Can you work these out from the model? Positions are in its coordinate system, mm. A direction names the side the tool comes from. Give positions to 0.01 mm unless a question says otherwise; leave off trailing zeros. Order: outer loops, then holes, each group sorted by start corner. A loop starts at its lowest first (then second) coordinate and runs counter-clockwise, first axis right, second up. Notation, with made-up numbers: M -21,67 L -7,67 A10 ccw -7,72 Z; hole C 65,34 d11. An arc over 180 degrees is marked long. One line per question, with ' | ' between items. Start each with the question number.
1) If we section it at C-C, the plane z = -25.4: Please give me the cut outline in (x, y) (3 decimals).
2) For faces 1 (the flat face through (84.16, 17.485, -14.31)), 2 (the flat face through (82.55, 12, -38)), which set-ups out of +Z, -Z, +X, -X, +Y, -Y let a thin tool reach every point of the face, with its end or its side?
3) If we section it at A-A, the plane x = 6.35: Please give me the cut outline in (y, z) (3 decimals), plus the area to 3 significant figures.
4) Please list where these lines run through material, in increasing order: line 1 along X through (y, z) = (1.5, -50.8); line 2 along X through (y, z) = (1, -25.4); line 3 along X through (y, z) = (4.5, -28.5) (3 decimals). Write a range as [from, to].
5) I'm going to push flat-ended pins straight in: pin 1 Ø4 at (y, z) = (11.5, -52.5) entering from -X; pin 2 Ø4.5 at (x, z) = (38.1, -25.4) entering from -Y; pin 3 Ø8.5 at (x, z) = (69.85, -50.8) entering from +Y (3 decimals). Where does each tip first touch, or does it pass through?
6) Thinking about a two-plate mould opening in Y: for faces 3 (the cylindrical face through (84.12, 11.27, -23.15)), 4 (the flat face through (84.16, 17.44, -61.935)), 5 (the cylindrical face through (7.151, 1.61, -22.856)), which applies, +Y half, -Y half, draft (parallel to the pull), parting line (faces both ways), or undercut?
7) If we section it at D-D, the plane z = -45: Please give me the cut outline in (x, y) (3 decimals).
8) If we section it at B-B, the plane y = 12.7: Please give me the cut outline in (x, z) (3 decimals).
```python
from build123d import *

# Parameters (mm, degrees)
SKETCH1_W               = 81.788
SKETCH1_H               = 63.5
BOSS_EXTRUDE1_DEPTH     = 3.175
EDGE_FLANGE1_DEPTH      = 63.5
SKETCH6_R               = 2.667
CUT_EXTRUDE1_DEPTH      = 108.856577222
SKETCH7_R               = 2.667
CUT_EXTRUDE2_DEPTH      = 106.875658203
CUT_EXTRUDE3_DEPTH      = 108.856577222
CUT_EXTRUDE3_DEPTH_BACK = 108.856577222
SKETCH8_W               = 104.248957023
SKETCH8_H               = 23.686680931
CHAMFER2_SIZE           = 3.175


# Sheet-metal steps are written as plain solids
with BuildPart() as part:
    # Sketch1 → Boss-Extrude1 (new body)
    with BuildSketch(Plane(origin=(0, 0, 0), x_dir=(1, 0, 0), z_dir=(0, 1, 0))):
        with Locations((40.894, 31.75)):
            Rectangle(SKETCH1_W, SKETCH1_H)
    extrude(amount=BOSS_EXTRUDE1_DEPTH)

    # Edge-Flange1 section (across the edge) → Edge-Flange1 (add)
    with BuildSketch(Plane(origin=(82.55, 3.175, 0), x_dir=(-1, 0, 0), z_dir=(0, 0, -1))):
        with BuildLine():
            Line((-3.175, 0.762), (-3.175, 15.875))
            Line((-3.175, 15.875), (0, 15.875))
            Line((0, 15.875), (0, 0.762))
            ThreePointArc((0, 0.762), (0.223184633, 0.223184633), (0.762, 0))
            Line((0.762, 0), (0.762, -3.175))
            ThreePointArc((0.762, -3.175), (-2.021879398, -2.021879398), (-3.175, 0.762))
        make_face()
    extrude(amount=EDGE_FLANGE1_DEPTH)

    # Sketch6 → Cut-Extrude1 (cut, through all)
    with BuildSketch(Plane(origin=(0, 3.175, 0), x_dir=(1, 0, 0), z_dir=(0, 1, 0))):
        with Locations(Location((6.35, 50.8, 0), (0, 0, 270))):
            Circle(SKETCH6_R)
        with Locations(Location((6.35, 25.4, 0), (0, 0, 270))):
            Circle(SKETCH6_R)
        with Locations((6.35, 0)):
            Circle(SKETCH6_R)
        with Locations(Location((69.85, 50.8, 0), (0, 0, 270))):
            Circle(SKETCH6_R)
        with Locations(Location((69.85, 25.4, 0), (0, 0, 270))):
            Circle(SKETCH6_R)
        with Locations((69.85, 0)):
            Circle(SKETCH6_R)
        with Locations(Location((38.1, 50.8, 0), (0, 0, 270))):
            Circle(SKETCH6_R)
        with Locations((38.1, 0)):
            Circle(SKETCH6_R)
        with Locations(Location((38.1, 25.4, 0), (0, 0, 270))):
            Circle(SKETCH6_R)
    extrude(amount=-CUT_EXTRUDE1_DEPTH, mode=Mode.SUBTRACT)

    # Sketch7 → Cut-Extrude2 (cut, through all)
    with BuildSketch(Plane.ZY.offset(-82.55)):
        with Locations(Location((-50.8, 12.7, 0), (0, 0, 270))):
            Circle(SKETCH7_R)
        with Locations(Location((-25.4, 12.7, 0), (0, 0, 270))):
            Circle(SKETCH7_R)
        with Locations((0, 12.7)):
            Circle(SKETCH7_R)
    extrude(amount=-CUT_EXTRUDE2_DEPTH, mode=Mode.SUBTRACT)

    # Sketch8 → Cut-Extrude3 (cut, two sides: drawn at the far end of the back side and taken through both)
    with BuildSketch(Plane(origin=(0, 3.175, 0), x_dir=(1, 0, 0), z_dir=(0, 1, 0)).offset(-CUT_EXTRUDE3_DEPTH_BACK)):
        with Locations((42.695076622, 0.856659535)):
            Rectangle(SKETCH8_W, SKETCH8_H)
    extrude(amount=CUT_EXTRUDE3_DEPTH + CUT_EXTRUDE3_DEPTH_BACK, mode=Mode.SUBTRACT)

    # Chamfer2
    chamfer2_edges = [part.edges().sort_by_distance(p)[0] for p in [
        (84.1375, 19.05, -12.7),
        (0, 1.5875, -12.7),
        (84.1375, 19.05, -63.5),
        (0, 1.5875, -63.5),
    ]]
    chamfer(chamfer2_edges, length=CHAMFER2_SIZE)


solid = part.part
```
Results found:
1) outline: M 0,0 L 3.683,0 L 3.683,3.175 L 0,3.175 Z; M 9.017,0 L 35.433,0 L 35.433,3.175 L 9.017,3.175 Z; M 40.767,0 L 67.183,0 L 67.183,3.175 L 40.767,3.175 Z; M 72.517,0 L 81.788,0 A3.937 ccw 85.725,3.937 L 85.725,10.033 L 82.55,10.033 L 82.55,3.937 A0.762 cw 81.788,3.175 L 72.517,3.175 Z; M 82.55,15.367 L 85.725,15.367 L 85.725,19.05 L 82.55,19.05 Z
2) face 1: +Z, +X, -X, +Y | face 2: +Z, -Z, -X, +Y
3) outline: M 0,-63.5 L 3.175,-63.5 L 3.175,-53.467 L 0,-53.467 Z; M 0,-48.133 L 3.175,-48.133 L 3.175,-28.067 L 0,-28.067 Z; M 0,-22.733 L 3.175,-22.733 L 3.175,-12.7 L 0,-12.7 Z | area: 127 mm²
4) line 1: x = [0, 3.68], [9.02, 35.43], [40.77, 67.18], [72.52, 84.88] | line 2: x = [0, 3.68], [9.02, 35.43], [40.77, 67.18], [72.52, 84.41] | line 3: x = [82.55, 85.725]
5) pin 1: stops at x = 82.55 | pin 2: passes through | pin 3: stops at y = 3.175
6) face 3: undercut | face 4: +Y half | face 5: draft
7) outline: M 0,0 L 81.788,0 A3.937 ccw 85.725,3.937 L 85.725,19.05 L 82.55,19.05 L 82.55,3.937 A0.762 cw 81.788,3.175 L 0,3.175 Z
8) outline: M 82.55,-63.5 L 85.725,-63.5 L 85.725,-53.467 L 82.55,-53.467 Z; M 82.55,-48.133 L 85.725,-48.133 L 85.725,-28.067 L 82.55,-28.067 Z; M 82.55,-22.733 L 85.725,-22.733 L 85.725,-12.7 L 82.55,-12.7 Z
